Autodesk Inventor part; units mm, degrees
ref_plane "YZ Plane" through (0, 0, 0) normal (1, 0, 0) x (0, 1, 0)
ref_plane "XZ Plane" through (0, 0, 0) normal (0, 1, 0) x (-1, 0, 0)
ref_plane "XY Plane" through (0, 0, 0) normal (0, 0, 1) x (1, 0, 0)
sketch "Sketch1" plane through (0, 0, 0) normal (0, 0, 1) x (1, 0, 0)
  circle A0 centre (0, 0) radius 11
  circle A1 centre (0, 84) radius 14 construction
  circle A2 centre (0, 0) radius 72 construction
  circle A3 centre (0, 84) radius 12 construction
  line L0 (0, 84) -> (0, 0) construction
  line L1 (-67.6579, 24.6255) -> (0, 0) construction
  line L2 (67.6579, 24.6255) -> (0, 0) construction
  circle A4 centre (0, 84) radius 35 construction
  line L3 (-60, 71.9226) -> (-60, 144) construction
  line L4 (-60, 144) -> (60, 144) construction
  line L5 (60, 144) -> (60, 71.9226) construction
  circle A5 centre (0, 0) radius 27.5
  line L6 (25.3583, -10.6399) -> (60, 71.9226) construction
  line L7 (-60, 71.9226) -> (-25.3583, -10.6399) construction
  line L8 (0, 0) -> (135.9462, -63.3927) construction
  line L9 (-24.7487, 59.2513) -> (24.7487, 59.2513) construction
  circle A6 centre (0, 84) radius 60 construction
  arc A7 (67.6579, 24.6255) -> (-67.6579, 24.6255) centre (0, 0) ccw
  arc A8 (66.9531, 24.3689) -> (-66.9531, 24.3689) centre (0, 0) ccw
  line L10 (67.3977, 25.3289) -> (67.4014, 25.3302)
  circle A9 centre (135.9462, -63.3927) radius 2
  circle A10 centre (135.9462, -63.3927) radius 7
  line L11 (-67.6579, 24.6255) -> (0, 0)
  line L12 (0, 0) -> (67.6579, 24.6255)
  line L13 (-8.1067, -26.2779) -> (133.8826, -70.0817)
  line L14 (139.7438, -57.5124) -> (14.9192, 23.1013)
  point P0 (24.7487, 108.7487)
  point P1 (-24.7487, 108.7487)
  point P2 (-25.8415, 9.4056)
  point P3 (32.419, 11.7996)
  point P4 (66.9531, 24.3689)
  point P5 (-66.9531, 24.3689)
  dimension "d7" = 70
  dimension "d2" = 24
  dimension "d3" = 144
  dimension "d4" = 28
  dimension "d5" = 22
  dimension "d6" = 220
  dimension "d8" = 360
  dimension "d9" = 55
  dimension "d10" = 150
  dimension "d11" = 45
  dimension "d12" = 120
  dimension "d13" = 0.75
  dimension "d14" = 4
  dimension "d15" = 14
extrude "Extrusion1" add sketch "Sketch1" along normal blind 30 contours A0 L12 A5 L11 | A0 L11 A5 L12 | L12 L14 A10 L13 A5 | A5 L14 L12 | L11 A8 L12 L14 A5 | A10
fillet "Fillet1" radius 6 2 edges at (-25.8415, 9.4056, 15) (32.419, 11.7996, 15)
equation "\"d3\" = 6 * d2"
properties part number "RT_ARM_MC_008_Capstand_Arm"
Input: part model. Units: mm. Frame: model coordinates. A direction names the side the tool comes from. Give positions to 0.01 mm unless a question says otherwise; leave off trailing zeros. Write each loop counter-clockwise with the first axis right and the second up, starting at its lowest first coordinate (ties: lowest second). Pieces come first, ordered by that corner, then holes.
Q1. Set-up query: faces 1 (the face through (37, 1, 30)), 2 (the face through (91.83, -26.57, 14.79)). Return all of +Z, -Z, +X, -X, +Y, -Y with unobstructed straight access to the full face (end or side cutting, diameter ignored); none if empty.
Q2. Section B-B, the plane y = 2.5. Output: boundary loops of the cut face in (x, z).
Q3. Pull-direction query (Y, two-part tool) for faces 3 (the face through (-2.38, 10.74, 14.79)), 4 (the face through (61.89, -47.87, 14.79)), 5 (the face through (-1.22, 71.24, 14.79)), 6 (the face through (142.35, -66.22, 14.79)); classes: pulls with the +Y half, pulls with the -Y half, needs draft (parallel to the pull), parting line crosses it, or undercut.
Q4. Section D-D, the plane y = 19. Output: boundary loops of the cut face in (x, z).
Q5. Section C-C, the plane z = 8.5. Output: boundary loops of the cut face in (x, y), plus the area to 3 significant figures.
Q6. First-contact query: P1, Ø10, axis at y = -30, z = 7.5, coming from the -X side; P2, Ø2, axis at y = 31, z = 4, coming from the -X side; P3, Ø4, axis at x = 47.5, z = 25.5, coming from the -Y side. Flat tips, straight axial feed; report the tip coordinate or a pass-through.
Q7. Material intervals for probe 1 along X at (y, z) = (-7, 25); probe 2 along X at (y, z) = (0, 17.75); probe 3 along X at (y, z) = (24.5, 24.5), sorted ascending.
Q8. Section A-A, the plane x = 55. Output: boundary loops of the cut face in (y, z), plus the area to 3 significant figures.
Filled in:
1. face 1: +Z, +X, -X, +Y, -Y
1. face 2: +Z, -Z, +X
2. outline: (-27.39, 0) - (-10.71, 0) - (-10.71, 30) - (-27.39, 30) - close; (10.71, 0) - (46.82, 0) - (46.82, 30) - (10.71, 30) - close
3. face 3: undercut
3. face 4: pulls with the -Y half
3. face 5: pulls with the +Y half
3. face 6: parting line crosses it
4. outline: (-52.2, 0) - (52.2, 0) - (52.2, 30) - (-52.2, 30) - close
5. outline: (-66.95, 24.37) - (-30.97, 11.27) arc R6 cw to (-27.11, 4.63) arc R27.5 ccw to (-8.11, -26.28) - (133.88, -70.08) arc R7 ccw to (139.74, -57.51) - (42.56, 5.25) arc R6 cw to (43.76, 15.93) - (66.95, 24.37) arc R71.25 ccw to start; hole circle Ø22 at (0, 0); hole circle Ø4 at (135.95, -63.39)
5. area: 11,400 mm2
6. P1: stops at x = -11.46
6. P2: stops at x = -64.63
6. P3: stops at y = -44.05
7. probe 1: x = -26.59 to -8.49, 8.49 to 61.53
7. probe 2: x = -27.5 to -11, 11 to 50.69
7. probe 3: x = -66.91 to 66.91
8. outline: (-45.75, 0) - (-2.78, 0) - (-2.78, 30) - (-45.75, 30) - close; (20.02, 0) - (45.29, 0) - (45.29, 30) - (20.02, 30) - close
8. area: 2,050 mm2
